from build123d import *

# Parameters (mm, degrees)
SKETCH1_W                                      = 152.4
SKETCH1_H                                      = 152.4
BOSS_EXTRUDE1_DEPTH                            = 12.7
F_1_4_20_TAPPED_HOLE1_D                        = 5.1054
CBORE_FOR_4_SOCKET_HEAD_CAP_SCREW1_D           = 3.2639
CBORE_FOR_4_SOCKET_HEAD_CAP_SCREW1_CBORE_D     = 5.55752
CBORE_FOR_4_SOCKET_HEAD_CAP_SCREW1_CBORE_DEPTH = 2.8448
F_2_56_TAPPED_HOLE1_D                          = 1.778
F_2_56_TAPPED_HOLE1_DEPTH                      = 5.7404
F_2_56_TAPPED_HOLE1_TIP                        = 0.53416509
F_2_56_TAPPED_HOLE2_D                          = 1.778
F_2_56_TAPPED_HOLE2_DEPTH                      = 5.7404
F_2_56_TAPPED_HOLE2_TIP                        = 0.53416509
CBORE_SLOT_FOR_4_SOCKET_HEAD_CAP_SCREW1_DEPTH  = 12.7
CBORE_START                                    = 9.8552
CBORE_SLOT_FOR_4_SOCKET_HEAD_CAP_SC_3_DEPTH    = 2.8448
CBORE_START_2                                  = 6.35
CBORE_SLOT_FOR_1_4_SOCKET_HEAD_CAP_SCREW_DEPTH = 6.35
CBORE_SLOT_FOR_1_4_SOCKET_HEAD_CAP_S_3_DEPTH   = 6.35


# Read off the part's stored shape, not the designer's step: CBORE SLOT for #4 Socket Head Cap Screw1, CBORE SLOT for 1/4 Socket Head Cap Screw3
with BuildPart() as part:
    # Sketch1 → Boss-Extrude1 (new body)
    with BuildSketch(Plane.XY):
        Rectangle(SKETCH1_W, SKETCH1_H)
    extrude(amount=BOSS_EXTRUDE1_DEPTH)

    # 1/4-20 Tapped Hole1 (through all)
    with Locations(Plane.XY.offset(12.7)):
        with Locations((44.45, 44.45), (44.45, -44.45), (-44.45, -44.45), (-44.45, 44.45)):
            Hole(F_1_4_20_TAPPED_HOLE1_D / 2)

    # CBORE for #4 Socket Head Cap Screw1 (through all)
    with Locations(Plane.XY.offset(12.7)):
        with Locations((-73.025, 63.5), (-73.025, 73.025), (73.025, 63.5), (73.025, 73.025), (73.025, -63.5), (73.025, -73.025), (-73.025, -63.5), (-73.025, -73.025)):
            CounterBoreHole(CBORE_FOR_4_SOCKET_HEAD_CAP_SCREW1_D / 2, CBORE_FOR_4_SOCKET_HEAD_CAP_SCREW1_CBORE_D / 2, CBORE_FOR_4_SOCKET_HEAD_CAP_SCREW1_CBORE_DEPTH)

    # #2-56 Tapped Hole1
    with Locations(Plane(origin=(0, 0, 0), x_dir=(-1, 0, 0), z_dir=(0, 0, -1))):
        with Locations((-63.5, -63.5), (-63.5, -34.163), (-29.083, -63.5), (-29.083, -34.163)):
            Hole(F_2_56_TAPPED_HOLE1_D / 2, depth=F_2_56_TAPPED_HOLE1_DEPTH)
            with Locations((0, 0, -(F_2_56_TAPPED_HOLE1_DEPTH + F_2_56_TAPPED_HOLE1_TIP / 2))):  # 118° drill point
                Cone(0, F_2_56_TAPPED_HOLE1_D / 2, F_2_56_TAPPED_HOLE1_TIP, mode=Mode.SUBTRACT)

    # #2-56 Tapped Hole2
    with Locations(Plane(origin=(0, 0, 0), x_dir=(-1, 0, 0), z_dir=(0, 0, -1))):
        with Locations((-63.5, 6.5278), (-63.5, 63.5), (-29.3878, 63.5), (-29.3878, 6.5278)):
            Hole(F_2_56_TAPPED_HOLE2_D / 2, depth=F_2_56_TAPPED_HOLE2_DEPTH)
            with Locations((0, 0, -(F_2_56_TAPPED_HOLE2_DEPTH + F_2_56_TAPPED_HOLE2_TIP / 2))):  # 118° drill point
                Cone(0, F_2_56_TAPPED_HOLE2_D / 2, F_2_56_TAPPED_HOLE2_TIP, mode=Mode.SUBTRACT)

    # CBORE SLOT for _4 Socket Head Cap Sc 2 → CBORE SLOT for #4 Socket Head Cap Screw1 (cut)
    with BuildSketch(Plane.XY):
        with BuildLine():
            Line((6.78815, 30.11805), (16.22425, 30.11805))
            ThreePointArc((16.22425, 30.11805), (17.8562, 31.75), (16.22425, 33.38195))
            Line((16.22425, 33.38195), (6.78815, 33.38195))
            ThreePointArc((6.78815, 33.38195), (5.1562, 31.75), (6.78815, 30.11805))
        make_face()
        with BuildLine():
            Line((6.78815, 11.06805), (16.22425, 11.06805))
            ThreePointArc((16.22425, 11.06805), (17.8562, 12.7), (16.22425, 14.33195))
            Line((16.22425, 14.33195), (6.78815, 14.33195))
            ThreePointArc((6.78815, 14.33195), (5.1562, 12.7), (6.78815, 11.06805))
        make_face()
    extrude(amount=CBORE_SLOT_FOR_4_SOCKET_HEAD_CAP_SCREW1_DEPTH, mode=Mode.SUBTRACT)

    # CBORE SLOT for _4 Socket Head Cap Sc 3 o → CBORE SLOT for _4 Socket Head Cap Sc 3 (cut)
    # profile 1 of 2: a face of its own
    with BuildSketch(Plane.XY.offset(CBORE_START)):
        with BuildLine():
            Line((6.78815, 28.97124), (16.22425, 28.97124))
            ThreePointArc((16.22425, 28.97124), (19.00301, 31.75), (16.22425, 34.52876))
            Line((16.22425, 34.52876), (6.78815, 34.52876))
            ThreePointArc((6.78815, 34.52876), (4.00939, 31.75), (6.78815, 28.97124))
        make_face()
        with BuildLine():
            ThreePointArc((16.22425, 33.38195), (17.8562, 31.75), (16.22425, 30.11805))
            Line((16.22425, 30.11805), (6.78815, 30.11805))
            ThreePointArc((6.78815, 30.11805), (5.1562, 31.75), (6.78815, 33.38195))
            Line((6.78815, 33.38195), (16.22425, 33.38195))
        make_face(mode=Mode.SUBTRACT)
    # profile 2 of 2: a face of its own
    with BuildSketch(Plane.XY.offset(CBORE_START)):
        with BuildLine():
            Line((6.78815, 9.92124), (16.22425, 9.92124))
            ThreePointArc((16.22425, 9.92124), (19.00301, 12.7), (16.22425, 15.47876))
            Line((16.22425, 15.47876), (6.78815, 15.47876))
            ThreePointArc((6.78815, 15.47876), (4.00939, 12.7), (6.78815, 9.92124))
        make_face()
        with BuildLine():
            ThreePointArc((16.22425, 14.33195), (17.8562, 12.7), (16.22425, 11.06805))
            Line((16.22425, 11.06805), (6.78815, 11.06805))
            ThreePointArc((6.78815, 11.06805), (5.1562, 12.7), (6.78815, 14.33195))
            Line((6.78815, 14.33195), (16.22425, 14.33195))
        make_face(mode=Mode.SUBTRACT)
    extrude(amount=CBORE_SLOT_FOR_4_SOCKET_HEAD_CAP_SC_3_DEPTH, mode=Mode.SUBTRACT)

    # CBORE SLOT for 1_4 Socket Head Cap S 2 → CBORE SLOT for 1/4 Socket Head Cap Screw3 (cut)
    with BuildSketch(Plane.XY.offset(CBORE_START_2)):
        with BuildLine():
            Line((-39.52875, -18.4658), (-39.52875, -12.5222))
            ThreePointArc((-39.52875, -12.5222), (-45.085, -6.96595), (-50.64125, -12.5222))
            Line((-50.64125, -12.5222), (-50.64125, -18.4658))
            ThreePointArc((-50.64125, -18.4658), (-45.085, -24.02205), (-39.52875, -18.4658))
        make_face()
        with BuildLine():
            Line((-20.47875, -18.4658), (-20.47875, -12.5222))
            ThreePointArc((-20.47875, -12.5222), (-26.035, -6.96595), (-31.59125, -12.5222))
            Line((-31.59125, -12.5222), (-31.59125, -18.4658))
            ThreePointArc((-31.59125, -18.4658), (-26.035, -24.02205), (-20.47875, -18.4658))
        make_face()
    extrude(amount=CBORE_SLOT_FOR_1_4_SOCKET_HEAD_CAP_SCREW_DEPTH, mode=Mode.SUBTRACT)

    # CBORE SLOT for 1_4 Socket Head Cap S 3 o → CBORE SLOT for 1_4 Socket Head Cap S 3 (cut)
    with BuildSketch(Plane.XY):
        with BuildLine():
            Line((-41.7068, -18.4658), (-41.7068, -12.5222))
            ThreePointArc((-41.7068, -12.5222), (-45.085, -9.144), (-48.4632, -12.5222))
            Line((-48.4632, -12.5222), (-48.4632, -18.4658))
            ThreePointArc((-48.4632, -18.4658), (-45.085, -21.844), (-41.7068, -18.4658))
        make_face()
        with BuildLine():
            Line((-22.6568, -18.4658), (-22.6568, -12.5222))
            ThreePointArc((-22.6568, -12.5222), (-26.035, -9.144), (-29.4132, -12.5222))
            Line((-29.4132, -12.5222), (-29.4132, -18.4658))
            ThreePointArc((-29.4132, -18.4658), (-26.035, -21.844), (-22.6568, -18.4658))
        make_face()
    extrude(amount=CBORE_SLOT_FOR_1_4_SOCKET_HEAD_CAP_S_3_DEPTH, mode=Mode.SUBTRACT)


solid = part.part
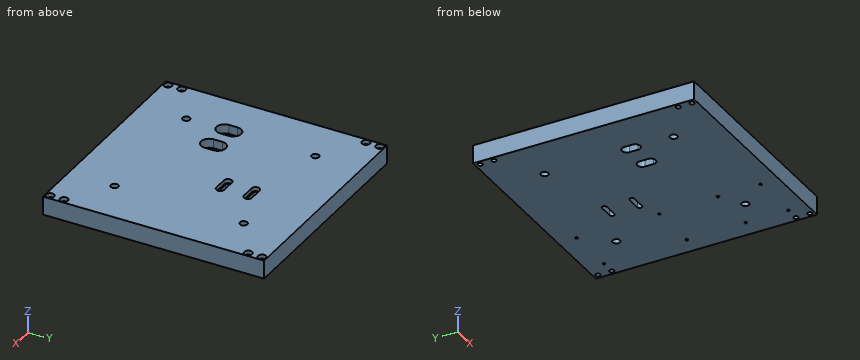
Source: CAD feature listing. Evaluate the final solid. Frame: model axes, mm. Give positions to 0.01 mm unless a question says otherwise; leave off trailing zeros. Loops run counter-clockwise (first coordinate to the right, second up) from the corner with the lowest first, then second, coordinate; pieces in that order, holes last. Notation, with made-up numbers: (37, -25) -> (49, -25) arc R20 cw to (49, -14) -> close; hole circle Ø10 at (71.5, -33.75). An arc over 180 degrees is marked (long way). Use a Markdown table: item, result. Add a question column.
1) Line query: line 1 along X through (y, z) = (-17.5, 10.25); line 2 along X through (y, z) = (44.5, 7.5). Output: solid intervals per line, ascending. Write a range as [from, to].
2) Section query C-C, the plane z = 3.75. Count the separate pieces of the cut face and the enclosed holes in it, then the cut area to 3 significant figures.
3) First-contact query: pin 1 (3 mm diameter, centred on x = -44.45, y = -44.45, fed in from +Z); pin 2 (1.7 mm diameter, centred on x = -73, y = -72, fed in from +Z). Flat tips, straight axial feed; report the tip coordinate or a pass-through.
4) Section query A-A, the plane y = 44.45. Return the cut outline in (x, z), then the cut area to 3 significant figures.
Numbers:
| question | item | result |
|---|---|---|
| 1 | line 1 | x = [-76.2, -50.64], [-39.53, -31.59], [-20.48, 76.2] |
| 1 | line 2 | x = [-76.2, -47], [-41.9, 41.9], [47, 76.2] |
| 2 | separate pieces | 1 |
| 2 | enclosed holes | 24 |
| 2 | area | 22,800 mm2 |
| 3 | pin 1 | passes through |
| 3 | pin 2 | stops at z = 9.86 |
| 4 | outline | (-76.2, 0) -> (-47, 0) -> (-47, 12.7) -> (-76.2, 12.7) -> close; (-41.9, 0) -> (41.9, 0) -> (41.9, 12.7) -> (-41.9, 12.7) -> close; (47, 0) -> (76.2, 0) -> (76.2, 12.7) -> (47, 12.7) -> close |
| 4 | area | 1,810 mm2 |
